Part model, mm, in its own coordinate system. Give positions to 0.01 mm unless a question says otherwise; leave off trailing zeros. Write each loop counter-clockwise with the first axis right and the second up, starting at its lowest first coordinate (ties: lowest second). Pieces come first, ordered by that corner, then holes. Notation, with made-up numbers: M 53,75 L 65,75 A26 ccw 65,114 Z; hole C 56.25,-10.5 d9. An arc over 180 degrees is marked long. Use a Markdown table: item, result.
```python
from build123d import *

# Parameters (mm, degrees)
F1_DEPTH = 2
F2_R     = 12.7
F3_R     = 2.54
F4_R     = 5.08


with BuildPart() as f1:
    # F0 (on Front) → F1 (new body)
    with BuildSketch(Plane.XZ):
        Polygon((-60.4972, 15), (-60.4972, 0), (60.5028, 0), (60.5028, 15), (7.4943, 35), (-7.5057, 35), align=None)
    extrude(amount=F1_DEPTH)

    # F2
    f2_edges = [f1.edges().sort_by_distance(p)[0] for p in [
        (-60.4972, -1, 15),
        (60.5028, -1, 15),
    ]]
    fillet(f2_edges, radius=F2_R)

    # F3
    f3_edges = [f1.edges().sort_by_distance(p)[0] for p in [
        (-60.4972, -1, 0),
        (60.5028, -1, 0),
    ]]
    fillet(f3_edges, radius=F3_R)

    # F4
    f4_edges = [f1.edges().sort_by_distance(p)[0] for p in [
        (-7.5057, -1, 35),
        (7.4943, -1, 35),
    ]]
    fillet(f4_edges, radius=F4_R)


solid = f1.part
```
1. Cut at C-C, the plane x = -25.5. Give the cut face in (y, z).
Findings below:
| item | result |
|---|---|
| outline | M -2,0 L 0,0 L 0,28.21 L -2,28.21 Z |
2. Drop a flat-ended pin along its axis: P1, Ø1, axis at x = 40, y = -1, coming from the +Z side. Give the stop position or say it passes through.
Findings below:
| item | result |
|---|---|
| P1 | z = 22.92 |
3. Cut at A-A, the plane y = -0.7. Give the cut face in (x, z).
Findings below:
| item | result |
|---|---|
| outline | M -60.5,2.54 A2.54 ccw -57.96,0 L 57.96,0 A2.54 ccw 60.5,2.54 L 60.5,6.22 A12.7 ccw 52.29,18.1 L 8.36,34.67 A5.08 ccw 6.57,35 L -6.58,35 A5.08 ccw -8.37,34.67 L -52.28,18.1 A12.7 ccw -60.5,6.22 Z |
4. Cut at B-B, the plane z = 14. Give the cut face in (x, y), then the cut area to 3 significant figures.
Findings below:
| item | result |
|---|---|
| outline | M -57.83,-2 L 57.84,-2 L 57.84,0 L -57.83,0 Z |
| area | 231 mm2 |
5. Drill centre lines: L1, parallel to Z at x = 36, y = -0.95; L2, parallel to Z at x = 31.5, y = -0.75; L3, parallel to X at y = -1.6, z = 13. Where is each one in solid material? Low to high.
Findings below:
| item | result |
|---|---|
| L1 | 0 to 24.24 |
| L2 | 0 to 25.94 |
| L3 | -58.54 to 58.54 |
